Autodesk Inventor part; units mm, degrees
ref_plane "YZ Plane" through (0, 0, 0) normal (1, 0, 0) x (0, 1, 0)
ref_plane "XZ Plane" through (0, 0, 0) normal (0, 1, 0) x (-1, 0, 0)
ref_plane "XY Plane" through (0, 0, 0) normal (0, 0, 1) x (1, 0, 0)
sketch "Sketch1" plane through (0, 0, 0) normal (0, 1, 0) x (-1, 0, 0)
  line L0 (-12.7, 12.7) -> (12.7, 12.7)
  line L1 (12.7, 12.7) -> (12.7, -12.7)
  line L2 (12.7, -12.7) -> (-12.7, -12.7)
  line L3 (-12.7, -12.7) -> (-12.7, 12.7)
  line L4 (-12.7, 12.7) -> (12.7, -12.7) construction
  line L5 (12.7, 12.7) -> (-12.7, -12.7) construction
  circle A0 centre (0, 0) radius 50
  line L6 (12.8, -7.7) -> (16.8, -7.7)
  line L7 (16.8, -7.7) -> (16.8, 7.7)
  line L8 (16.8, 7.7) -> (12.8, 7.7)
  line L9 (12.8, 7.7) -> (12.8, -7.7)
  line L10 (-12.5, -17.7) -> (12.5, -17.7) construction
  line L11 (12.5, -17.7) -> (12.5, -42.7) construction
  line L12 (12.5, -42.7) -> (-12.5, -42.7) construction
  line L13 (-12.5, -42.7) -> (-12.5, -17.7) construction
  line L14 (0, -12.7) -> (0, -17.7) construction
  line L15 (17.8, 12.5) -> (42.8, 12.5) construction
  line L16 (42.8, 12.5) -> (42.8, -12.5) construction
  line L17 (42.8, -12.5) -> (17.8, -12.5) construction
  line L18 (17.8, -12.5) -> (17.8, 12.5) construction
  line L19 (-42.7, 12.5) -> (-17.7, 12.5) construction
  line L20 (-17.7, 12.5) -> (-17.7, -12.5) construction
  line L21 (-17.7, -12.5) -> (-42.7, -12.5) construction
  line L22 (-42.7, -12.5) -> (-42.7, 12.5) construction
  line L23 (-12.5, 42.7) -> (12.5, 42.7) construction
  line L24 (12.5, 42.7) -> (12.5, 17.7) construction
  line L25 (12.5, 17.7) -> (-12.5, 17.7) construction
  line L26 (-12.5, 17.7) -> (-12.5, 42.7) construction
  line L27 (17.8, 0) -> (12.8, 0) construction
  line L28 (-12.7, 0) -> (-17.7, 0) construction
  line L29 (0, 17.7) -> (0, 12.7) construction
  point P0 (30.3, 12.5)
  point P1 (-30.2, 12.5)
  point P2 (0, 42.7)
  dimension "d0" = 25.4
  dimension "d1" = 25.4
  dimension "d2" = 0.1
  dimension "d3" = 4
  dimension "d4" = 100
  dimension "d7" = 5
  dimension "d8" = 5
  dimension "d21" = 25
  dimension "d28" = 25
  dimension "d35" = 25
  dimension "d44" = 25
  dimension "d73" = 5
  dimension "d74" = 5
  dimension "d75" = 5
  dimension "d76" = 5
extrude "Extrusion1" add sketch "Sketch1" against normal blind 20 contours L0 L1 L2 L3 | A0 | L9 L8 L7 L6
extrude "Extrusion2" add sketch "Sketch1" along normal blind 1 contours L9 L8 L7 L6
pattern_circular "Circular Pattern1" count 4 over 360 about axis through (0, 0, 0) along (0, -1, 0) of "Extrusion2"
decal "Decal1"
decal "Decal2"
decal "Decal3"
decal "Decal4"
equation "\"d8\" = d7"
equation "\"d73\" = d74"
equation "\"d75\" = d74"
equation "\"d76\" = d74"
properties part number "Spin Chuck"
Source: CAD feature listing. Evaluate the final solid. Frame: model axes, mm. Give positions to 0.01 mm unless a question says otherwise; leave off trailing zeros. Order: outer loops, then holes, each group sorted by start corner. A loop starts at its lowest first (then second) coordinate and runs counter-clockwise, first axis right, second up. Notation, with made-up numbers: (78.25, -4) -> (133.25, -4) arc R36 cw to (133.25, 34) -> close; hole circle Ø6 at (76, -20.75). An arc over 180 degrees is marked (long way). Use a Markdown table: item, result.
Q1. Section B-B (x = 0). Return the cut outline in (y, z), and give its area (3 significant figures).
A:
| item | result |
|---|---|
| outline | (-20, -50) -> (0, -50) -> (0, -16.8) -> (1, -16.8) -> (1, -12.8) -> (0, -12.8) -> (0, 12.8) -> (1, 12.8) -> (1, 16.8) -> (0, 16.8) -> (0, 50) -> (-20, 50) -> close |
| area | 2,010 mm^2 |
Q2. Section C-C (y = -17.75). Return the cut outline in (x, z), and give its area (3 significant figures).
A:
| item | result |
|---|---|
| outline | circle Ø100 at (0, 0) |
| area | 7,850 mm^2 |
Q3. First-contact query: P1, Ø3, axis at y = -13, z = -2.5, coming from the +X side; P2, Ø0.8, axis at y = 0.5, z = -14.5, coming from the +X side; P3, Ø0.8, axis at y = 0.5, z = 2, coming from the -X side. Flat tips, straight axial feed; report the tip coordinate or a pass-through.
A:
| item | result |
|---|---|
| P1 | x = 49.99 |
| P2 | x = 7.7 |
| P3 | x = -16.8 |
Q4. Section D-D (x = 37.5). Return the cut outline in (y, z).
A:
| item | result |
|---|---|
| outline | (-20, -33.07) -> (0, -33.07) -> (0, 33.07) -> (-20, 33.07) -> close |
Q5. Section A-A (z = 0). Return the cut outline in (x, y).
A:
| item | result |
|---|---|
| outline | (-50, -20) -> (50, -20) -> (50, 0) -> (16.8, 0) -> (16.8, 1) -> (12.8, 1) -> (12.8, 0) -> (-12.8, 0) -> (-12.8, 1) -> (-16.8, 1) -> (-16.8, 0) -> (-50, 0) -> close |
Q6. Material intervals for line 1 (Y direction, x = 5.5, z = -23); line 2 (X direction, y = -6, z = 39); line 3 (X direction, y = -12.75, z = 38), sorted ascending. Write a range as [from, to].
A:
| item | result |
|---|---|
| line 1 | [-20, 0] |
| line 2 | [-31.29, 31.29] |
| line 3 | [-32.5, 32.5] |
